Design review of the part built by this model. Coordinates are the model's own, in mm. Face numbers are marked on the shaded views. A direction names the side the tool comes from. Coordinates: 2 decimals unless noted, no trailing zeros. Loops run counter-clockwise (first coordinate to the right, second up) from the corner with the lowest first, then second, coordinate; pieces in that order, holes last. Notation, with made-up numbers: (34, -23.5) -> (54, -23.5) arc R23 cw to (54, -3.5) -> close; hole circle Ø8 at (45.5, 71). An arc over 180 degrees is marked (long way). One line per item, written item: value. Start each with the question number.
1. Add section A-A on z = 2.75. Write out the cut boundary in (x, y).
2. Machinability: for the marked faces 5, 6 and 7, which of the approach directions +Z, -Z, +X, -X, +Y, -Y give a long, thin tool a straight path to every point of the face, cutting with its end or side? Answer none if there is none.
3. Insertion check: pin 1 (1 mm diameter, centred on x = 17.5, z = 0.5, fed in from -Y); pin 2 (1 mm diameter, centred on x = 19, z = 1.5, fed in from +Y). Each pin has a flat end and moves straight along its axis. Give the tip position at first contact, or say it passes through.
4. For probe 1 along Y at (x, z) = (17.5, 2.55); probe 2 along X at (y, z) = (5.25, 0.8); probe 3 along Y at (x, z) = (15.5, 1.5), list the stretches that pass through material, from the lowest coordinate up.
5. Add section B-B on x = 18.75. Write out the cut boundary in (y, z), plus the area to 3 significant figures.
6. Add section D-D on x = 19.75. Write out the cut boundary in (y, z).
7. Add section C-C on y = 1.25. Write out the cut boundary in (x, z), plus the area to 3 significant figures.
8. Draft analysis for pull direction X (two halves, no side actions). For the marked faces 1, 2, 3 and 4, state which applies: pulls with the +X half, pulls with the -X half, needs draft (parallel to the pull), parting line crosses it, or undercut.
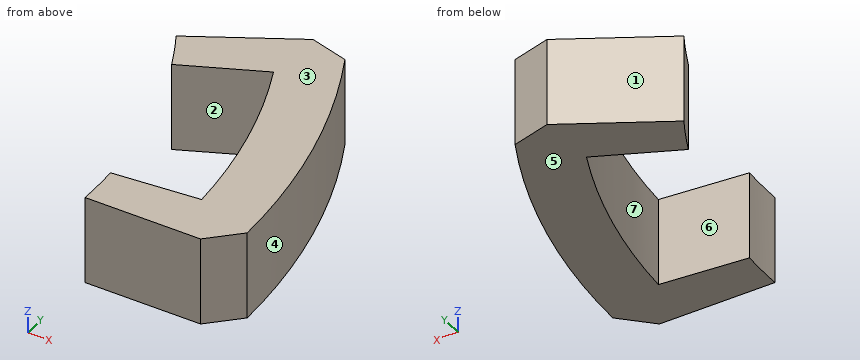
```python
from build123d import *

# Parameters (mm, degrees)
CYLINDER001_W            = 17
CYLINDER001_H            = 3
CYLINDER001_ANGLE        = 30
CYLINDER_W               = 20
CYLINDER_H               = 3
CYLINDER_ANGLE           = 20
CYLINDER_PLACEMENT_ANGLE = 5
CYLINDER002_W            = 22
CYLINDER002_H            = 3
CYLINDER002_ANGLE        = 30
CHAMFER007003_SIZE       = 1


with BuildPart() as cylinder001:
    # Cylinder001 → Cylinder001 (revolve)
    with BuildSketch(Plane.XZ):
        with Locations((8.5, 1.5)):
            Rectangle(CYLINDER001_W, CYLINDER001_H)
    revolve(axis=Axis((0, 0, 0), (0, 0, 1)), revolution_arc=CYLINDER001_ANGLE)


with BuildPart() as cylinder:
    # Cylinder → Cylinder (revolve)
    with BuildSketch(Plane.XZ):
        with Locations((10, 1.5)):
            Rectangle(CYLINDER_W, CYLINDER_H)
    revolve(axis=Axis((0, 0, 0), (0, 0, 1)), revolution_arc=CYLINDER_ANGLE)


with BuildPart() as cylinder_1:
    # Cylinder placement: moved
    add(cylinder.part.rotate(Axis((0, 0, 0), (0, 0, 1)), CYLINDER_PLACEMENT_ANGLE))


with BuildPart() as chamfer007003:
    # Cylinder002 → Cylinder002 (revolve)
    with BuildSketch(Plane.XZ):
        with Locations((11, 1.5)):
            Rectangle(CYLINDER002_W, CYLINDER002_H)
    revolve(axis=Axis((0, 0, 0), (0, 0, 1)), revolution_arc=CYLINDER002_ANGLE)

    # Cut001: cut Cylinder
    add(cylinder_1.part, mode=Mode.SUBTRACT)

    # Cut002: cut Cylinder001
    add(cylinder001.part, mode=Mode.SUBTRACT)

    # Chamfer007003
    chamfer007003_edges = [chamfer007003.edges().sort_by_distance(p)[0] for p in [
        (19.052559, 11, 1.5),
        (22, 0, 1.5),
    ]]
    chamfer(chamfer007003_edges, length=CHAMFER007003_SIZE)


solid = chamfer007003.part
```
Worked answers:
1. outline: (14.72, 8.5) arc R17 cw to (15.41, 7.18) -> (18.13, 8.45) arc R20 cw to (19.92, 1.74) -> (16.94, 1.48) arc R17 cw to (17, 0) -> (21, 0) -> (21.98, 1) arc R22 ccw to (19.53, 10.12) -> (18.19, 10.5) -> close
2. face 5: -Z, +X, -X, +Y, -Y
2. face 6: +Z, -Z, -X
2. face 7: +Z, -Z
3. pin 1: stops at y = 0
3. pin 2: stops at y = 10.41
4. probe 1: y = 0 to 1.53, 8.16 to 10.1
4. probe 2: x = 19.3 to 21.36
4. probe 3: y = 7.23 to 8.95
5. outline: (0, 0) -> (1.64, 0) -> (1.64, 3) -> (0, 3) -> close; (6.96, 0) -> (10.34, 0) -> (10.34, 3) -> (6.96, 3) -> close
5. area: 15.1 mm²
6. outline: (0, 0) -> (1.73, 0) -> (1.73, 3) -> (0, 3) -> close; (3.15, 0) -> (9.69, 0) -> (9.69, 3) -> (3.15, 3) -> close
7. outline: (16.95, 0) -> (21.96, 0) -> (21.96, 3) -> (16.95, 3) -> close
7. area: 15.0 mm²
8. face 1: pulls with the -X half
8. face 2: undercut
8. face 3: needs draft
8. face 4: pulls with the +X half
